For this review, take the finished solid that the model builds, in its own axes (mm). Face numbers are marked on the shaded views. A direction names the side the tool comes from. Coordinates: 2 decimals unless noted, no trailing zeros. Loops run counter-clockwise (first coordinate to the right, second up) from the corner with the lowest first, then second, coordinate; pieces in that order, holes last. Notation, with made-up numbers: M -28,54 L 14,54 A20 ccw 14,68 Z; hole C 16.5,-22.5 d3. An arc over 180 degrees is marked long. Write item = value, one per line.
from build123d import *

# Parameters (mm, degrees)
SKETCH1_R           = 4
BOSS_EXTRUDE1_DEPTH = 30
SKETCH2_R           = 1.5
CUT_EXTRUDE1_DEPTH  = 30


with BuildPart() as part:
    # Sketch1 → Boss-Extrude1 (new body)
    with BuildSketch(Plane.XY):
        Polygon((-16, -7), (-9, -7), (-5, -11), (5, -11), (9, -7), (16, -7), (16, 5), (17, 5), (17, 11), (7, 11), (7, 10), (-7, 10), (-7, 11), (-17, 11), (-17, 5), (-16, 5), align=None)
        Circle(SKETCH1_R, mode=Mode.SUBTRACT)
    extrude(amount=BOSS_EXTRUDE1_DEPTH)

    # Sketch2 → Cut-Extrude1 (cut)
    with BuildSketch(Plane(origin=(0, 11, 0), x_dir=(-1, 0, 0), z_dir=(0, 1, 0))):
        with Locations(Location((12, 24, 0), (0, 0, 90))):
            Circle(SKETCH2_R)
        with Locations(Location((12, 6, 0), (0, 0, 90))):
            Circle(SKETCH2_R)
        with Locations(Location((-12, 24, 0), (0, 0, 90))):
            Circle(SKETCH2_R)
        with Locations(Location((-12, 6, 0), (0, 0, 90))):
            Circle(SKETCH2_R)
    extrude(amount=-CUT_EXTRUDE1_DEPTH, mode=Mode.SUBTRACT)


solid = part.part
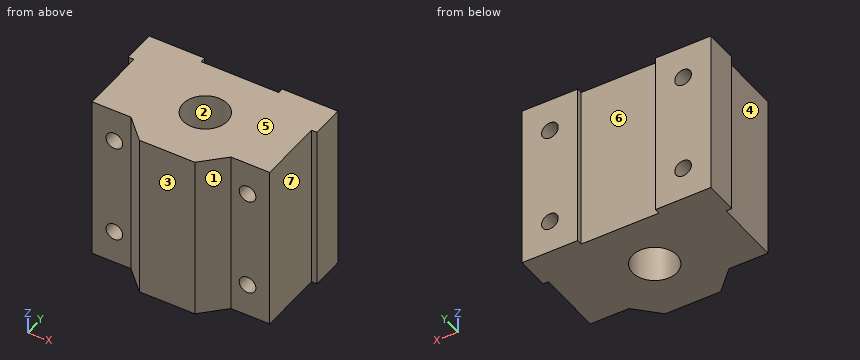
Q1. Add section D-D (y = 4.5). Write out the cut boundary in (x, z).
Solved:
outline = M -16,0 L 16,0 L 16,30 L -16,30 Z; hole C -12,6 d3; hole C -12,24 d3; hole C 12,6 d3; hole C 12,24 d3
Q2. Machinability: for the marked faces 4, 5, 6 and 7, which of the approach directions +Z, -Z, +X, -X, +Y, -Y give a long, thin tool a straight path to every point of the face, cutting with its end or side? Answer none if there is none.
Solved:
face_4 = +Z, -Z, -X, -Y
face_5 = +Z, +X, -X, +Y, -Y
face_6 = +Z, -Z, +Y
face_7 = +Z, -Z, +X, -Y
Q3. Add section A-A (y = 0). Write out the cut boundary in (x, z), and give its area (3 significant figures).
Solved:
outline = M -16,0 L -4,0 L -4,30 L -16,30 Z; M 4,0 L 16,0 L 16,30 L 4,30 Z; hole C -12,6 d3; hole C -12,24 d3; hole C 12,6 d3; hole C 12,24 d3
area = 692 mm²
Q4. Add section B-B (z = 6). Write out the cut boundary in (x, y).
Solved:
outline = M -17,5 L -16,5 L -16,-7 L -13.5,-7 L -13.5,11 L -17,11 Z; M -10.5,-7 L -9,-7 L -5,-11 L 5,-11 L 9,-7 L 10.5,-7 L 10.5,11 L 7,11 L 7,10 L -7,10 L -7,11 L -10.5,11 Z; M 13.5,-7 L 16,-7 L 16,5 L 17,5 L 17,11 L 13.5,11 Z; hole C 0,0 d8
Q5. Add section C-C (x = 0). Write out the cut boundary in (y, z), and give its area (3 significant figures).
Solved:
outline = M -11,0 L -4,0 L -4,30 L -11,30 Z; M 4,0 L 10,0 L 10,30 L 4,30 Z
area = 390 mm²
Q6. For pin 1 Ø2 at (x, z) = (-11, 14) entering from -Y; pin 2 Ø3 at (x, z) = (9.5, 17) entering from -Y; pin 3 Ø3.5 at (y, z) = (2, 19.5) entering from +X, all flat-tipped, find the tip position at first contact; note any pin that passes through.
Solved:
pin_1 = -7
pin_2 = -8
pin_3 = 16
Q7. For line 1 along Y through (x, z) = (0, 15.75); line 2 along X through (y, z) = (-3.5, 7.25); line 3 along X through (y, z) = (1, 6), list the stretches that pass through material, from the lowest coordinate up.
Solved:
line_1 = -11 to -4, 4 to 10
line_2 = -16 to -12.83, -11.17 to -1.94, 1.94 to 11.17, 12.83 to 16
line_3 = -16 to -13.5, -10.5 to -3.87, 3.87 to 10.5, 13.5 to 16
Q8. Draft analysis for pull direction X (two halves, no side actions). For the marked faces 1, 2 and 3, state which applies: +X half, -X half, draft (parallel to the pull), parting line (faces both ways), or undercut.
Solved:
face_1 = +X half
face_2 = undercut
face_3 = draft
